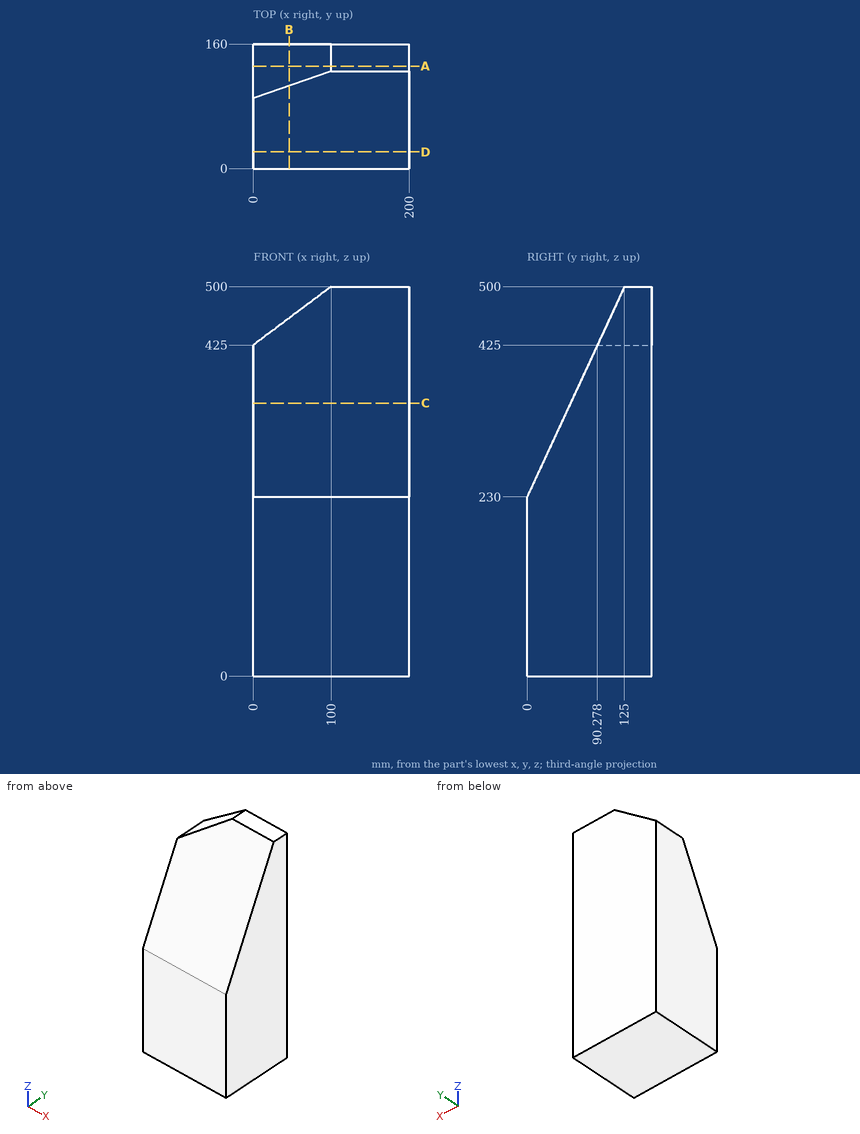
Drawing for the job (mm, zero at the part's lowest x, y, z). Round coordinates to 2 decimals unless told otherwise and drop trailing zeros. Write each loop counter-clockwise with the first axis right and the second up, starting at its lowest first coordinate (ties: lowest second). Pieces come first, ordered by that corner, then holes. Notation, with made-up numbers: M 65,34 L 85,34 A24 ccw 85,57 Z; hole C 78.5,44.5 d6. An arc over 180 degrees is marked long. Answer in a Markdown table with one row per item.
1. Saw through at B-B (x = 46). List the corners of the cut face in (y, z), and give its area (3 significant figures).
Geometry check:
| item | result |
|---|---|
| outline | M 0,0 L 160,0 L 160,459.5 L 106.25,459.5 L 0,230 Z |
| area | 61,300 mm2 |
2. Saw through at A-A (y = 131.5). List the corners of the cut face in (x, z), and give its area (4 significant figures).
Geometry check:
| item | result |
|---|---|
| outline | M 0,0 L 200,0 L 200,500 L 100,500 L 0,425 Z |
| area | 96,250 mm2 |
3. Saw through at D-D (y = 21.5). List the corners of the cut face in (x, z), and give its area (3 significant figures).
Geometry check:
| item | result |
|---|---|
| outline | M 0,0 L 200,0 L 200,276.44 L 0,276.44 Z |
| area | 55,300 mm2 |
4. Saw through at C-C (z = 350.5). List the corners of the cut face in (x, y).
Geometry check:
| item | result |
|---|---|
| outline | M 0,55.79 L 200,55.79 L 200,160 L 0,160 Z |
5. Probe L1, parallel to Z at x = 191, y = 71; L2, parallel to Y at x = 59, z = 314; L3, parallel to Y at x = 123, z = 384. List the from-to ranges inside material, lowest first. Write a range as [from, to].
Geometry check:
| item | result |
|---|---|
| L1 | [0, 383.36] |
| L2 | [38.89, 160] |
| L3 | [71.3, 160] |
